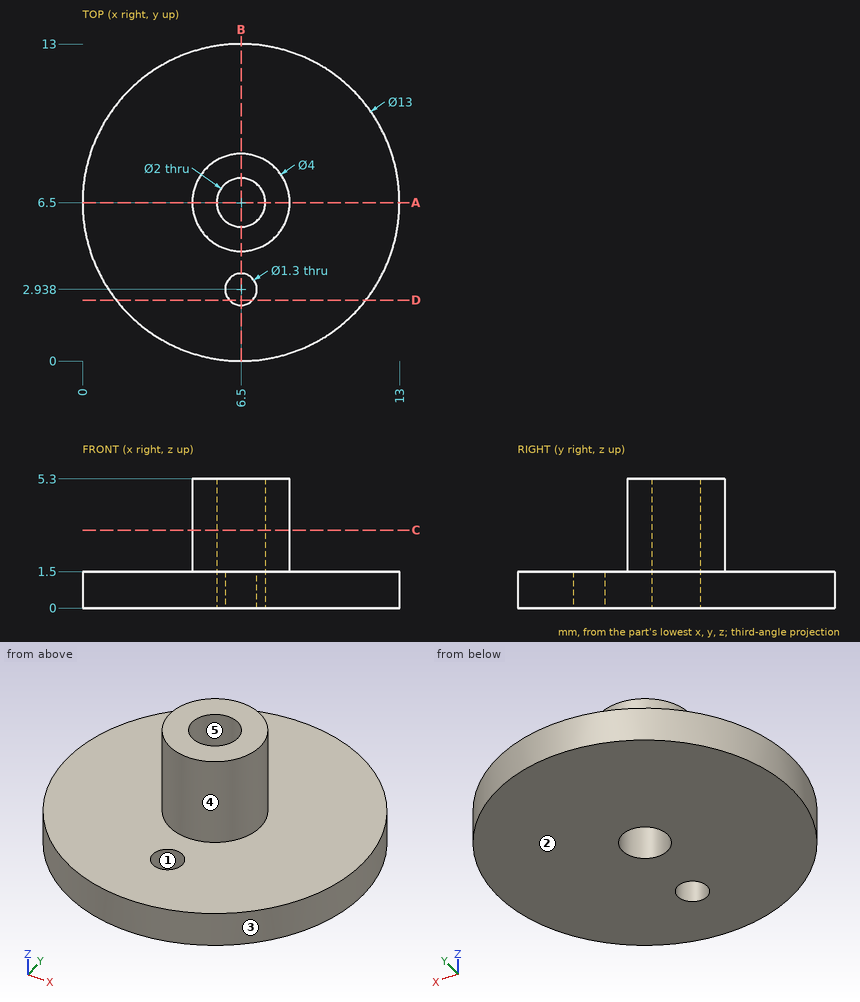
Geometry check sheet. Reference: drawing and pictorial views, mm from the part's lowest x, y, z. A direction names the side the tool comes from. Give positions to 0.01 mm unless a question says otherwise; leave off trailing zeros. Write each loop counter-clockwise with the first axis right and the second up, starting at its lowest first coordinate (ties: lowest second). Pieces come first, ordered by that corner, then holes.
Item 1: Cross-section at D-D (y = 2.5). Enter the section's corners in (x, z).
Item 2: Cross-section at A-A (y = 6.5). Enter the section's corners in (x, z).
Item 3: Gauge pin test, flat ends, axial feed: pin 1 (3 mm diameter, centred on x = 3.5, y = 3, fed in from +Z); pin 2 (2 mm diameter, centred on x = 10.5, z = 4.5, fed in from -Y); pin 3 (2 mm diameter, centred on y = 2, z = 2, fed in from -X). Record the tip position at first contact, or that the pin passes through.
Item 4: Cross-section at C-C (z = 3.2). Enter the section's corners in (x, y).
Item 5: Draft check along Y on the marked faces 1, 2 and 3. Enter one of: released by +Y, released by -Y, zero draft, split by the parting line, or undercut.
Item 6: Scan lines: L1, parallel to Y at x = 6.5, z = 2.9; L2, parallel to Z at x = 8.25, y = 2.5. Record each from-to range of solid material in increasing order.
Item 7: Access from +Z, -Z, +X, -X, +Y, -Y to the whole of each face (thin tool, end or side, straight path). Record for the marked faces 4 and 5.
Item 8: Cross-section at B-B (x = 6.5). Enter the section's corners in (y, z).
Report:
1. outline: (1.38, 0) - (6.02, 0) - (6.02, 1.5) - (1.38, 1.5) - close; (6.98, 0) - (11.62, 0) - (11.62, 1.5) - (6.98, 1.5) - close
2. outline: (0, 0) - (5.5, 0) - (5.5, 5.3) - (4.5, 5.3) - (4.5, 1.5) - (0, 1.5) - close; (7.5, 0) - (13, 0) - (13, 1.5) - (8.5, 1.5) - (8.5, 5.3) - (7.5, 5.3) - close
3. pin 1: stops at z = 1.5
3. pin 2: passes through
3. pin 3: stops at x = 1.11
4. outline: circle Ø4 at (6.5, 6.5); hole circle Ø2 at (6.5, 6.5)
5. face 1: undercut
5. face 2: zero draft
5. face 3: split by the parting line
6. L1: y = 4.5 to 5.5, 7.5 to 8.5
6. L2: z = 0 to 1.5
7. face 4: +Z
7. face 5: +Z, -Z
8. outline: (0, 0) - (2.29, 0) - (2.29, 1.5) - (0, 1.5) - close; (3.59, 0) - (5.5, 0) - (5.5, 5.3) - (4.5, 5.3) - (4.5, 1.5) - (3.59, 1.5) - close; (7.5, 0) - (13, 0) - (13, 1.5) - (8.5, 1.5) - (8.5, 5.3) - (7.5, 5.3) - close
